from build123d import *

# Parameters (mm, degrees)
SK_MAIN_EXTRUSION_R  = 3.4
MAIN_EXTRUSION_DEPTH = 25


with BuildPart() as part:
    # Sk Main Extrusion → Main Extrusion (new body)
    with BuildSketch(Plane.XY):
        with BuildLine():
            Line((4.190076845, -16.671180212), (5.222054351, -19.506515107))
            ThreePointArc((5.222054351, -19.506515107), (5.496641489, -19.864364033), (5.926823816, -20))
            Line((5.926823816, -20), (18.5, -20))
            ThreePointArc((18.5, -20), (19.560660172, -19.560660172), (20, -18.5))
            Line((20, -18.5), (20, -5.926823816))
            ThreePointArc((20, -5.926823816), (19.864364033, -5.496641489), (19.506515107, -5.222054351))
            Line((19.506515107, -5.222054351), (16.671180212, -4.190076845))
            ThreePointArc((16.671180212, -4.190076845), (16.563886241, -4.175951325), (16.460675177, -4.208493649))
            Line((16.460675177, -4.208493649), (15.111296024, -4.987558066))
            Line((15.111296024, -4.987558066), (14.845251581, -5.718509166))
            Line((14.845251581, -5.718509166), (15.81984631, -8.396186179))
            ThreePointArc((15.81984631, -8.396186179), (15.786489799, -8.811074612), (15.450654467, -9.056960151))
            ThreePointArc((15.450654467, -9.056960151), (12.665882372, -8.933433013), (10.272684887, -7.504160339))
            Line((10.272684887, -7.504160339), (9.309262274, -6.540737726))
            ThreePointArc((9.309262274, -6.540737726), (6.6, 0), (9.309262274, 6.540737726))
            Line((9.309262274, 6.540737726), (10.272684887, 7.504160339))
            ThreePointArc((10.272684887, 7.504160339), (12.665882372, 8.933433013), (15.450654467, 9.056960151))
            ThreePointArc((15.450654467, 9.056960151), (15.786489799, 8.811074612), (15.81984631, 8.396186179))
            Line((15.81984631, 8.396186179), (14.845251581, 5.718509166))
            Line((14.845251581, 5.718509166), (15.111296024, 4.987558066))
            Line((15.111296024, 4.987558066), (16.460675176, 4.208493649))
            ThreePointArc((16.460675176, 4.208493649), (16.563886241, 4.175951325), (16.671180212, 4.190076845))
            Line((16.671180212, 4.190076845), (19.506515107, 5.222054351))
            ThreePointArc((19.506515107, 5.222054351), (19.864364033, 5.496641489), (20, 5.926823816))
            Line((20, 5.926823816), (20, 18.5))
            ThreePointArc((20, 18.5), (19.560660172, 19.560660172), (18.5, 20))
            Line((18.5, 20), (5.926823816, 20))
            ThreePointArc((5.926823816, 20), (5.496641489, 19.864364033), (5.222054351, 19.506515107))
            Line((5.222054351, 19.506515107), (4.190076845, 16.671180212))
            ThreePointArc((4.190076845, 16.671180212), (4.175951325, 16.563886241), (4.208493649, 16.460675176))
            Line((4.208493649, 16.460675176), (4.987558066, 15.111296024))
            Line((4.987558066, 15.111296024), (5.718509166, 14.845251581))
            Line((5.718509166, 14.845251581), (8.396186179, 15.81984631))
            ThreePointArc((8.396186179, 15.81984631), (8.811074612, 15.786489799), (9.056960151, 15.450654467))
            ThreePointArc((9.056960151, 15.450654467), (8.933433013, 12.665882372), (7.504160339, 10.272684887))
            Line((7.504160339, 10.272684887), (6.540737726, 9.309262274))
            ThreePointArc((6.540737726, 9.309262274), (0, 6.6), (-6.540737726, 9.309262274))
            Line((-6.540737726, 9.309262274), (-7.504160339, 10.272684887))
            ThreePointArc((-7.504160339, 10.272684887), (-8.933433013, 12.665882372), (-9.056960151, 15.450654467))
            ThreePointArc((-9.056960151, 15.450654467), (-8.811074612, 15.786489799), (-8.396186179, 15.81984631))
            Line((-8.396186179, 15.81984631), (-5.718509166, 14.845251581))
            Line((-5.718509166, 14.845251581), (-4.987558066, 15.111296024))
            Line((-4.987558066, 15.111296024), (-4.208493649, 16.460675177))
            ThreePointArc((-4.208493649, 16.460675177), (-4.175951325, 16.563886241), (-4.190076845, 16.671180212))
            Line((-4.190076845, 16.671180212), (-5.222054351, 19.506515107))
            ThreePointArc((-5.222054351, 19.506515107), (-5.496641489, 19.864364033), (-5.926823816, 20))
            Line((-5.926823816, 20), (-18.5, 20))
            ThreePointArc((-18.5, 20), (-19.560660172, 19.560660172), (-20, 18.5))
            Line((-20, 18.5), (-20, 5.926823816))
            ThreePointArc((-20, 5.926823816), (-19.864364033, 5.496641489), (-19.506515107, 5.222054351))
            Line((-19.506515107, 5.222054351), (-16.671180212, 4.190076845))
            ThreePointArc((-16.671180212, 4.190076845), (-16.563886241, 4.175951325), (-16.460675177, 4.208493649))
            Line((-16.460675177, 4.208493649), (-15.111296024, 4.987558066))
            Line((-15.111296024, 4.987558066), (-14.845251581, 5.718509166))
            Line((-14.845251581, 5.718509166), (-15.81984631, 8.396186179))
            ThreePointArc((-15.81984631, 8.396186179), (-15.786489799, 8.811074612), (-15.450654467, 9.056960151))
            ThreePointArc((-15.450654467, 9.056960151), (-12.665882372, 8.933433013), (-10.272684887, 7.504160339))
            Line((-10.272684887, 7.504160339), (-9.309262274, 6.540737726))
            ThreePointArc((-9.309262274, 6.540737726), (-6.6, 0), (-9.309262274, -6.540737726))
            Line((-9.309262274, -6.540737726), (-10.272684887, -7.504160339))
            ThreePointArc((-10.272684887, -7.504160339), (-12.665882372, -8.933433013), (-15.450654467, -9.056960151))
            ThreePointArc((-15.450654467, -9.056960151), (-15.786489799, -8.811074612), (-15.81984631, -8.396186179))
            Line((-15.81984631, -8.396186179), (-14.845251581, -5.718509166))
            Line((-14.845251581, -5.718509166), (-15.111296024, -4.987558066))
            Line((-15.111296024, -4.987558066), (-16.460675177, -4.208493649))
            ThreePointArc((-16.460675177, -4.208493649), (-16.563886241, -4.175951325), (-16.671180212, -4.190076845))
            Line((-16.671180212, -4.190076845), (-19.506515107, -5.222054351))
            ThreePointArc((-19.506515107, -5.222054351), (-19.864364033, -5.496641489), (-20, -5.926823816))
            Line((-20, -5.926823816), (-20, -18.5))
            ThreePointArc((-20, -18.5), (-19.560660172, -19.560660172), (-18.5, -20))
            Line((-18.5, -20), (-5.926823816, -20))
            ThreePointArc((-5.926823816, -20), (-5.496641489, -19.864364033), (-5.222054351, -19.506515107))
            Line((-5.222054351, -19.506515107), (-4.190076845, -16.671180212))
            ThreePointArc((-4.190076845, -16.671180212), (-4.175951325, -16.563886241), (-4.208493649, -16.460675177))
            Line((-4.208493649, -16.460675177), (-4.987558066, -15.111296024))
            Line((-4.987558066, -15.111296024), (-5.718509166, -14.845251581))
            Line((-5.718509166, -14.845251581), (-8.396186179, -15.81984631))
            ThreePointArc((-8.396186179, -15.81984631), (-8.811074612, -15.786489799), (-9.056960151, -15.450654467))
            ThreePointArc((-9.056960151, -15.450654467), (-8.933433013, -12.665882372), (-7.504160339, -10.272684887))
            Line((-7.504160339, -10.272684887), (-6.540737726, -9.309262274))
            ThreePointArc((-6.540737726, -9.309262274), (0, -6.6), (6.540737726, -9.309262274))
            Line((6.540737726, -9.309262274), (7.504160339, -10.272684887))
            ThreePointArc((7.504160339, -10.272684887), (8.933433013, -12.665882372), (9.056960151, -15.450654467))
            ThreePointArc((9.056960151, -15.450654467), (8.811074612, -15.786489799), (8.396186179, -15.81984631))
            Line((8.396186179, -15.81984631), (5.718509166, -14.845251581))
            Line((5.718509166, -14.845251581), (4.987558066, -15.111296024))
            Line((4.987558066, -15.111296024), (4.208493649, -16.460675177))
            ThreePointArc((4.208493649, -16.460675177), (4.175951325, -16.563886241), (4.190076845, -16.671180212))
        make_face()
        Circle(SK_MAIN_EXTRUSION_R, mode=Mode.SUBTRACT)
    extrude(amount=-MAIN_EXTRUSION_DEPTH)


solid = part.part
Part model, mm, in its own coordinate system. A direction names the side the tool comes from. Coordinates: 2 decimals unless noted, no trailing zeros. Order: outer loops, then holes, each group sorted by start corner. A loop starts at its lowest first (then second) coordinate and runs counter-clockwise, first axis right, second up.
(1) Pin check, flat tip, straight feed: pin 1 Ø2 at (y, z) = (-2.5, -12.5) entering from +X. Stop position of the tip, or through.
Check sheet entries:
pin 1: stops at x = 7.29
(2) Pull direction X, two halves, no side cores. Call faces 4 (the face through (0.1, 6.6, -12.3)), 5 (the face through (12, -20, -12)), 6 (the face through (-18.109, 4.713, -12.325)): pulls with the +X half, pulls with the -X half, needs draft (parallel to the pull), parting line crosses it, or undercut.
Check sheet entries:
face 4: undercut
face 5: needs draft
face 6: pulls with the -X half
(3) Probe L1, parallel to Y at x = 14, z = -23; L2, parallel to Y at x = 0, z = -15.75; L3, parallel to X at y = -11.5, z = -7.5. List the from-to ranges inside material, lowest first.
Check sheet entries:
L1: y = -20 to -9.17, 9.17 to 20
L2: y = -6.6 to -3.4, 3.4 to 6.6
L3: x = -20 to -8.44, 8.44 to 20
(4) Tool access for faces 1 (the face through (0, 5, -25)), 2 (the face through (4.7, -18.07, -12.32)), 3 (the face through (15.34, 7.08, -12.32)): list every direction of +Z, -Z, +X, -X, +Y, -Y with a clear straight run to the whole face (end or side of a thin tool).
Check sheet entries:
face 1: -Z, +X, -X, +Y, -Y
face 2: +Z, -Z, -Y
face 3: +Z, -Z
(5) Slice it at A-A, the plane x = 0. Write the cut outline in (y, z), and give its area (3 significant figures).
Check sheet entries:
outline: (-6.6, -25) - (-3.4, -25) - (-3.4, 0) - (-6.6, 0) - close; (3.4, -25) - (6.6, -25) - (6.6, 0) - (3.4, 0) - close
area: 160 mm2
